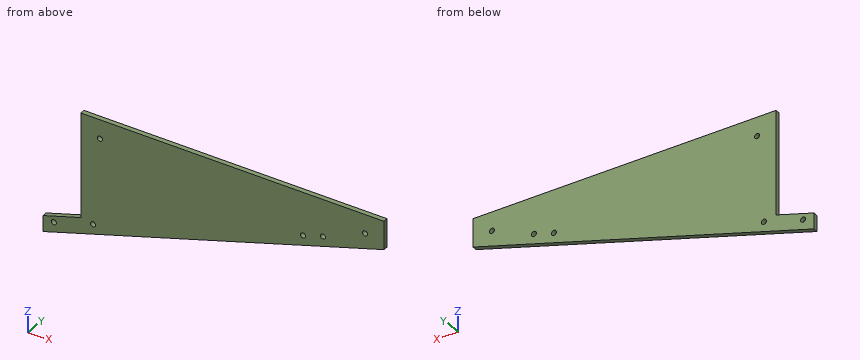
```python
from build123d import *

# Parameters (mm, degrees)
SKETCH1_R           = 3.429
BOSS_EXTRUDE1_DEPTH = 6.35
BOSS_EXTRUDE2_DEPTH = 6.35
CUT_EXTRUDE1_REACH  = 8.35
SKETCH3_R           = 3.429


with BuildPart() as part:
    # Sketch1 → Boss-Extrude1 (new body)
    with BuildSketch(Plane(origin=(0, 0, 0), x_dir=(1, 0, 0), z_dir=(0, 1, 0))):
        Polygon((0, 0), (406.4, 0), (406.4, 38.1), (0, 161.925), align=None)
        with Locations((381, 25.4)):
            Circle(SKETCH1_R, mode=Mode.SUBTRACT)
        with Locations((25.4, 25.4)):
            Circle(SKETCH1_R, mode=Mode.SUBTRACT)
    extrude(amount=BOSS_EXTRUDE1_DEPTH)

    # Sketch2 → Boss-Extrude2 (add)
    with BuildSketch(Plane(origin=(0, 6.35, 0), x_dir=(1, 0, 0), z_dir=(0, 1, 0))):
        Polygon((0, 161.925), (-50.8, 177.403125), (-50.8, 155.961232961), (0, 140.483107961), align=None)
    extrude(amount=-BOSS_EXTRUDE2_DEPTH)

    # Sketch3 → Cut-Extrude1 (cut, up to next)
    with BuildSketch(Plane(origin=(0, 6.35, 0), x_dir=(1, 0, 0), z_dir=(0, 1, 0)), mode=Mode.PRIVATE) as cut_extrude1_sk1:
        with Locations((324.672621663, 49.724892693)):
            Circle(SKETCH3_R)
    cut_extrude1_tool1 = extrude(cut_extrude1_sk1.sketch, amount=-CUT_EXTRUDE1_REACH, mode=Mode.PRIVATE) & part.part
    add(cut_extrude1_tool1.solids().sort_by_distance((324.672622, 6.35, -49.724893))[0], mode=Mode.SUBTRACT)
    # Sketch3 → Cut-Extrude1 (cut, up to next)
    with BuildSketch(Plane(origin=(0, 6.35, 0), x_dir=(1, 0, 0), z_dir=(0, 1, 0)), mode=Mode.PRIVATE) as cut_extrude1_sk2:
        with Locations((16.261590572, 143.693878729)):
            Circle(SKETCH3_R)
    cut_extrude1_tool2 = extrude(cut_extrude1_sk2.sketch, amount=-CUT_EXTRUDE1_REACH, mode=Mode.PRIVATE) & part.part
    add(cut_extrude1_tool2.solids().sort_by_distance((16.261591, 6.35, -143.693879))[0], mode=Mode.SUBTRACT)
    # Sketch3 → Cut-Extrude1 (cut, up to next)
    with BuildSketch(Plane(origin=(0, 6.35, 0), x_dir=(1, 0, 0), z_dir=(0, 1, 0)), mode=Mode.PRIVATE) as cut_extrude1_sk3:
        with Locations((297.810987833, 57.909296751)):
            Circle(SKETCH3_R)
    cut_extrude1_tool3 = extrude(cut_extrude1_sk3.sketch, amount=-CUT_EXTRUDE1_REACH, mode=Mode.PRIVATE) & part.part
    add(cut_extrude1_tool3.solids().sort_by_distance((297.810988, 6.35, -57.909297))[0], mode=Mode.SUBTRACT)
    # Sketch3 → Cut-Extrude1 (cut, up to next)
    with BuildSketch(Plane(origin=(0, 6.35, 0), x_dir=(1, 0, 0), z_dir=(0, 1, 0)), mode=Mode.PRIVATE) as cut_extrude1_sk4:
        with Locations((-36.278616697, 159.702223131)):
            Circle(SKETCH3_R)
    cut_extrude1_tool4 = extrude(cut_extrude1_sk4.sketch, amount=-CUT_EXTRUDE1_REACH, mode=Mode.PRIVATE) & part.part
    add(cut_extrude1_tool4.solids().sort_by_distance((-36.278617, 6.35, -159.702223))[0], mode=Mode.SUBTRACT)


solid = part.part
```
For this review, take the finished solid that the model builds, in its own axes (mm). Coordinates: 2 decimals unless noted, no trailing zeros. Loops run counter-clockwise (first coordinate to the right, second up) from the corner with the lowest first, then second, coordinate; pieces in that order, holes last. Notation, with made-up numbers: (63.25, 55.25) - (100.25, 55.25) arc R19 cw to (100.25, 77.25) - close; hole circle Ø1 at (52, 79.25). An arc over 180 degrees is marked (long way). Use one line per item in the form item = value. Start each with the question number.
1) Take a section at B-B (z = -104.5). State the section outline as (x, y) points.
2) To check wall thickness, follow probe 1 along X at (y, z) = (4.5, -25.4); probe 2 along Z at (x, y) = (381, 4); probe 3 along X at (y, z) = (5, -18.5). State the ranges of each line that lie inside material, in increasing order. Write a range as from..to.
3) For pin 1 (3 mm diameter, centred on x = 179.5, y = 2, fed in from -Z), flat-tipped, find the tip position at first contact; note if it passes through.
4) Take a section at C-C (x = 290). State the section outline as (y, z) points, plus the area to 3 significant figures.
5) Take a section at A-A (y = 1). State the section outline as (x, z) points, plus the area to 3 significant figures.
From the geometry:
q1.outline = (0, 0) - (188.47, 0) - (188.47, 6.35) - (0, 6.35) - close
q2.probe_1 = 0..21.97, 28.83..377.57, 384.43..406.4
q2.probe_2 = -45.84..-28.83, -21.97..0
q2.probe_3 = 0..406.4
q3.pin_1 = -107.69
q4.outline = (0, -73.57) - (6.35, -73.57) - (6.35, 0) - (0, 0) - close
q4.area = 467 mm2
q5.outline = (-50.8, -177.4) - (406.4, -38.1) - (406.4, 0) - (0, 0) - (0, -140.48) - (-50.8, -155.96) - close; hole circle Ø6.86 at (-36.28, -159.7); hole circle Ø6.86 at (16.26, -143.69); hole circle Ø6.86 at (25.4, -25.4); hole circle Ø6.86 at (297.81, -57.91); hole circle Ø6.86 at (324.67, -49.72); hole circle Ø6.86 at (381, -25.4)
q5.area = 41,500 mm2
